```python
from build123d import *

# Parameters (mm, degrees)
BOSS_EXTRUDE1_DEPTH = 4.7625
F_1_0_RADIUS_R      = 25.4
F_0_1_RADIUS_R      = 2.54
F_0_25_RADIUS_R     = 6.35
F_0_5_RADIUS_R      = 12.7
F_0_0625_RADIUS_R   = 1.5875


with BuildPart() as part:
    # Sketch1 → Boss-Extrude1 (new body)
    with BuildSketch(Plane.XY):
        Polygon((0, 0), (154.94, 0), (194.3735, 36.322), (206.1845, 36.322), (206.1845, 31.115), (224.5995, 31.115), (224.5995, 37.846), (211.6455, 50.8), (188.595, 50.8), (151.13, 26.9875), (3.81, 26.9875), (-33.655, 50.8), (-56.7055, 50.8), (-69.6595, 37.846), (-69.6595, 36.322), (-69.6595, 31.115), (-51.2445, 31.115), (-51.2445, 36.322), (-39.4335, 36.322), align=None)
    extrude(amount=BOSS_EXTRUDE1_DEPTH)

    # 1.0 Radius
    f_1_0_radius_edges = [part.edges().sort_by_distance(p)[0] for p in [
        (154.94, 0, 2.38125),
        (0, 0, 2.38125),
    ]]
    fillet(f_1_0_radius_edges, radius=F_1_0_RADIUS_R)

    # 0.1 Radius
    f_0_1_radius_edges = [part.edges().sort_by_distance(p)[0] for p in [
        (3.81, 26.9875, 2.38125),
        (151.13, 26.9875, 2.38125),
    ]]
    fillet(f_0_1_radius_edges, radius=F_0_1_RADIUS_R)

    # 0.25 Radius
    f_0_25_radius_edges = [part.edges().sort_by_distance(p)[0] for p in [
        (211.6455, 50.8, 2.38125),
        (194.3735, 36.322, 2.38125),
        (-39.4335, 36.322, 2.38125),
        (-56.7055, 50.8, 2.38125),
    ]]
    fillet(f_0_25_radius_edges, radius=F_0_25_RADIUS_R)

    # 0.5 Radius
    f_0_5_radius_edges = [part.edges().sort_by_distance(p)[0] for p in [
        (188.595, 50.8, 2.38125),
        (-33.655, 50.8, 2.38125),
    ]]
    fillet(f_0_5_radius_edges, radius=F_0_5_RADIUS_R)

    # 0.0625 Radius
    f_0_0625_radius_edges = [part.edges().sort_by_distance(p)[0] for p in [
        (206.1845, 36.322, 2.38125),
        (-51.2445, 36.322, 2.38125),
    ]]
    fillet(f_0_0625_radius_edges, radius=F_0_0625_RADIUS_R)


solid = part.part
```
Here's how the part is built. I have some questions about the finished solid (model axes, mm). A direction names the side the tool comes from. Give positions to 0.01 mm unless a question says otherwise; leave off trailing zeros. Write each loop counter-clockwise with the first axis right and the second up, starting at its lowest first coordinate (ties: lowest second). Pieces come first, ordered by that corner, then holes.
(1) Will these pins go through, and if not, where does the flat tip stop? pin 1 (1.4 mm diameter, centred on x = 217, z = 2, fed in from -Y) (3 decimals); pin 2 (6 mm diameter, centred on x = 168, y = 5.5, fed in from +Z) (3 decimals); pin 3 (5 mm diameter, centred on x = 114, y = 15, fed in from -Z); pin 4 (1.4 mm diameter, centred on x = 199.5, z = 2.5, fed in from -Y).
Output values:
pin 1: stops at y = 31.115
pin 2: passes through
pin 3: stops at z = 0
pin 4: stops at y = 36.32
(2) On a 3-axis mill with a long thin cutter (end or side, diameter ignored), from which of +Z, -Z, +X, -X, +Y, -Y can I reach the whole of each face in a straight line? I mean faces 1 (the face through (-46, 36.322, 2)), 2 (the face through (-13.44, 37.95, 2.35)), 3 (the face through (215, 31.115, 2)). Say none if no direction works.
Output values:
face 1: +Z, -Z, -Y
face 2: +Z, -Z, +Y
face 3: +Z, -Z, +X, -Y
(3) Imagine slicing it at B-B, the plane y = 45.5. Write out the boundary of the cut face in (x, z).
Output values:
outline: (-62.01, 0) - (-25.32, 0) - (-25.32, 4.76) - (-62.01, 4.76) - close; (180.26, 0) - (216.95, 0) - (216.95, 4.76) - (180.26, 4.76) - close
(4) If I drill on L1, parallel to X at y = 32.5, z = 3.55; L2, parallel to Y at x = 83.5, z = 1.4; L3, parallel to X at y = 31, z = 1.95, over which ranges is the centre line in solid material (lowest first)?
Output values:
L1: x = -69.66 to -51.24, -35.28 to -4.86, 159.8 to 190.22, 206.18 to 224.6
L2: y = 0 to 26.99
L3: x = -33.66 to -2.5, 157.44 to 188.6
(5) Imagine slicing it at D-D, the plane y = 14. Write out the boundary of the cut face in (x, z).
Output values:
outline: (-15.2, 0) - (170.14, 0) - (170.14, 4.76) - (-15.2, 4.76) - close
(6) Imagine slicing it at C-C, the plane x = 141. Write out the boundary of the cut face in (y, z), and give its area (3 significant figures).
Output values:
outline: (0, 0) - (26.99, 0) - (26.99, 4.76) - (0, 4.76) - close
area: 129 mm2
